Here's how the part is built. I have some questions about the finished solid (model axes, mm). Coordinates: 2 decimals unless noted, no trailing zeros. Loops run counter-clockwise (first coordinate to the right, second up) from the corner with the lowest first, then second, coordinate; pieces in that order, holes last. Notation, with made-up numbers: M 29,44 L 76,44 A11 cw 76,51 Z; hole C -7,27 d7. An arc over 180 degrees is marked long. Use one line per item in the form item = value. Start each with the question number.
(1) Please list where these lines run through material, in increasing order: L1, parallel to Y at x = 177.8, z = 4; L2, parallel to X at y = 8, z = 1.25; L3, parallel to Y at x = 33.5, z = 5.5.
(2) Imagine slicing it at D-D, the plane y = 31.5. Please give me the cut outline in (x, z).
(3) Imagine slicing it at A-A, the plane x = 177.8. Please give me the cut outline in (y, z).
(4) Imagine slicing it at B-B, the plane z = 4.5. Please give me the cut outline in (x, y).
(5) Imagine slicing it at C-C, the plane x = 112. Please give me the cut outline in (y, z), and give its area (3 significant figures).
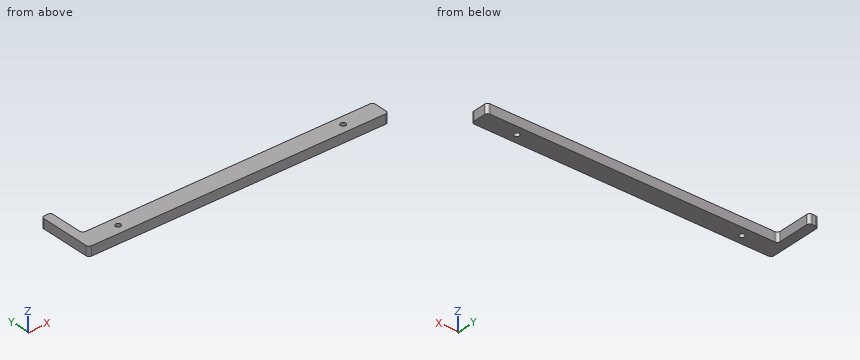
```python
from build123d import *

# Parameters (mm, degrees)
SKETCH2_W                 = 203.2
SKETCH2_H                 = 12.7
BOSS_EXTRUDE1_DEPTH       = 6.35
SKETCH3_W                 = 6.35
SKETCH3_H                 = 6.35
BOSS_EXTRUDE2_DEPTH       = 25.4
FILLET2_R                 = 2
F_6_CLEARANCE_HOLE1_D     = 3.6576
F_6_CLEARANCE_HOLE1_DEPTH = 10.16
F_6_CLEARANCE_HOLE1_TIP   = 1.0988539


with BuildPart() as part:
    # Sketch2 → Boss-Extrude1 (new body)
    with BuildSketch(Plane.XY):
        with Locations((101.6, 6.35)):
            Rectangle(SKETCH2_W, SKETCH2_H)
    extrude(amount=BOSS_EXTRUDE1_DEPTH)

    # Sketch3 → Boss-Extrude2 (add)
    with BuildSketch(Plane(origin=(0, 12.7, 0), x_dir=(1, 0, 0), z_dir=(0, 1, 0))):
        with Locations((3.175, -3.175)):
            Rectangle(SKETCH3_W, SKETCH3_H)
    extrude(amount=BOSS_EXTRUDE2_DEPTH)

    # Fillet2
    fillet2_edges = [part.edges().sort_by_distance(p)[0] for p in [
        (6.35, 12.7, 3.175),
        (0, 38.1, 3.175),
        (6.35, 38.1, 3.175),
        (203.2, 12.7, 3.175),
        (203.2, 0, 3.175),
        (0, 0, 3.175),
    ]]
    fillet(fillet2_edges, radius=FILLET2_R)

    # #6 Clearance Hole1
    with Locations(Plane.XY.offset(6.35)):
        with Locations((177.8, 6.35), (25.4, 6.35)):
            Hole(F_6_CLEARANCE_HOLE1_D / 2, depth=F_6_CLEARANCE_HOLE1_DEPTH)
            with Locations((0, 0, -(F_6_CLEARANCE_HOLE1_DEPTH + F_6_CLEARANCE_HOLE1_TIP / 2))):  # 118° drill point
                Cone(0, F_6_CLEARANCE_HOLE1_D / 2, F_6_CLEARANCE_HOLE1_TIP, mode=Mode.SUBTRACT)


solid = part.part
```
Answer:
q1.L1 = 0 to 4.52, 8.18 to 12.7
q1.L2 = 0 to 24.61, 26.19 to 177.01, 178.59 to 203.2
q1.L3 = 0 to 12.7
q2.outline = M 0,0 L 6.35,0 L 6.35,6.35 L 0,6.35 Z
q3.outline = M 0,0 L 4.52,0 L 4.52,6.35 L 0,6.35 Z; M 8.18,0 L 12.7,0 L 12.7,6.35 L 8.18,6.35 Z
q4.outline = M 0,2 A2 ccw 2,0 L 201.2,0 A2 ccw 203.2,2 L 203.2,10.7 A2 ccw 201.2,12.7 L 8.35,12.7 A2 cw 6.35,14.7 L 6.35,36.1 A2 ccw 4.35,38.1 L 2,38.1 A2 ccw 0,36.1 Z; hole C 25.4,6.35 d3.66; hole C 177.8,6.35 d3.66
q5.outline = M 0,0 L 12.7,0 L 12.7,6.35 L 0,6.35 Z
q5.area = 80.6 mm²
